Input: part model. Units: mm. Frame: model coordinates. Face numbers are marked on the shaded views. Coordinates: 2 decimals unless noted, no trailing zeros. Loops run counter-clockwise (first coordinate to the right, second up) from the corner with the lowest first, then second, coordinate; pieces in that order, holes last.
(1) Mould query, pull axis X, two halves, no side actions, for the marked faces 1, 2 and 3. Classes: released by +X, released by -X, zero draft, split by the parting line, or undercut.
(2) Section A-A, the plane x = -156. Return loops of the section in (y, z).
(3) Contact query for flat-ended pins moving along their axis: P1, Ø12, axis at x = -45, y = 86.5, coming from the +Z side; P2, Ø5, axis at x = -19, y = 39.5, coming from the +Z side; P3, Ø1.5, axis at x = -121.5, y = 24, coming from the +Z side; P4, Ø10, axis at y = 40.5, z = 27, coming from the +X side. Output: stop coordinate, or through.
(4) Line query: L1, parallel to Y at x = -132, z = 29.5; L2, parallel to Z at x = -169, y = 8.5; L3, parallel to Z at x = -155, y = 55. Output: solid intervals per line, ascending.
(5) Section C-C, the plane y = 38.5. Return loops of the section in (x, z).
(6) Section B-B, the plane y = 87.5. Return loops of the section in (x, z), then the cut area to 3 significant figures.
```python
from build123d import *

# Parameters (mm, degrees)
F1_DEPTH = 180
F2_W     = 60
F2_H     = 6
F2_H_2   = 20
F3_DEPTH = 5
F4_R     = 1
F5_DEPTH = 60
F6_DEPTH = 60


with BuildPart() as f1:
    # F0 (on Right) → F1 (new body)
    with BuildSketch(Plane.YZ):
        Polygon((105.484205862, 22.4625121504), (-4.515794138, 25.4625121504), (-4.515794138, 5.4625121504), (105.484205862, 5.4625121504), align=None)
    extrude(amount=-F1_DEPTH)

    # F2 (on face) → F3 (join)
    with BuildSketch(Plane.XZ.offset(4.515794138)):
        with Locations((-90, 28.4625121504)):
            Rectangle(F2_W, F2_H)
        with Locations((-90, 15.4625121504)):
            Rectangle(F2_W, F2_H_2)
    extrude(amount=F3_DEPTH)

    # F4
    f4_edges = [f1.edges().sort_by_distance(p)[0] for p in [
        (-90, -4.515794, 31.462512),
    ]]
    fillet(f4_edges, radius=F4_R)

    # F5 (add, through all): a face of the model
    f5_faces = [f1.faces().sort_by_distance(p)[0] for p in [
        (-60, -7.0195585786, 18.4413858238),
    ]]
    extrude(f5_faces, amount=F5_DEPTH)

    # F6 (add, through all): a face of the model
    f6_faces = [f1.faces().sort_by_distance(p)[0] for p in [
        (-120, -7.0195585786, 18.4413858238),
    ]]
    extrude(f6_faces, amount=F6_DEPTH)


solid = f1.part
```
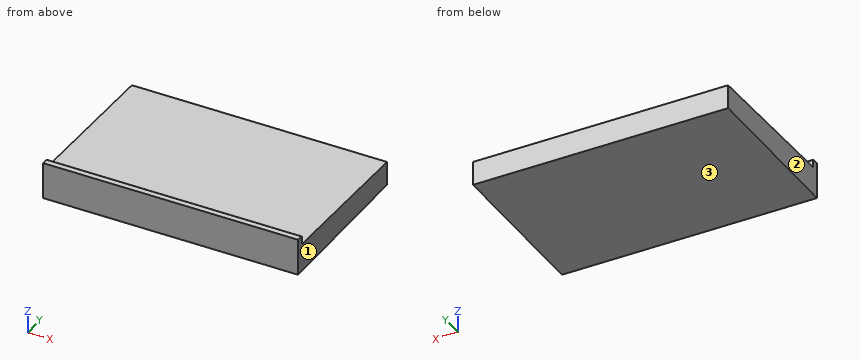
Report:
1. face 1: released by +X
1. face 2: released by -X
1. face 3: zero draft
2. outline: (-9.52, 5.46) - (105.48, 5.46) - (105.48, 22.46) - (-4.52, 25.46) - (-4.52, 30.46) arc R1 ccw to (-5.52, 31.46) - (-9.52, 31.46) - close
3. P1: stops at z = 23.14
3. P2: stops at z = 24.33
3. P3: stops at z = 24.71
3. P4: stops at x = 0
4. L1: y = -9.52 to -4.52
4. L2: z = 5.46 to 25.11
4. L3: z = 5.46 to 23.84
5. outline: (-180, 5.46) - (0, 5.46) - (0, 24.29) - (-180, 24.29) - close
6. outline: (-180, 5.46) - (0, 5.46) - (0, 22.95) - (-180, 22.95) - close
6. area: 3,150 mm2
